Build history of the part. All positions in model axes, mm. A direction names the side the tool comes from. Give positions to 0.01 mm unless a question says otherwise; leave off trailing zeros. Order: outer loops, then holes, each group sorted by start corner. A loop starts at its lowest first (then second) coordinate and runs counter-clockwise, first axis right, second up. Notation, with made-up numbers: (-16, -27) - (-2, -27) arc R8 cw to (-2, -13) - close; hole circle Ø2 at (-19.5, 45.5). An arc over 180 degrees is marked (long way). Write each question's results on one line, items separated by ' | '. Start each with the question number.
from build123d import *

# Parameters (mm, degrees)
PAD026_DEPTH    = 5
SKETCH058_R     = 2
POCKET036_DEPTH = 5.001
CHAMFER020_SIZE = 2


with BuildPart() as part:
    # Sketch053 → Pad026 (new body)
    with BuildSketch(Plane.XY):
        with BuildLine():
            Line((-81.323184, -45.417713), (-81.323184, -107.8))
            Line((-81.323184, -107.8), (-105.823184, -107.8))
            Line((-105.823184, -107.8), (-105.823184, 216.2))
            Line((-105.823184, 216.2), (-81.323184, 216.2))
            Line((-81.323184, 216.2), (-81.323184, -27.417713))
            Line((-89.323184, -27.417713), (-81.323184, -27.417713))
            ThreePointArc((-89.323184, -27.417713), (-98.323184, -36.417713), (-89.323184, -45.417713))
            Line((-89.323184, -45.417713), (-81.323184, -45.417713))
        make_face()
    extrude(amount=PAD026_DEPTH)

    # Sketch058 (on Face10 of Pad026) → Pocket036 (cut, through all)
    with BuildSketch(Plane.XY.offset(5)):
        with Locations((-99.573184, 211.2)):
            Circle(SKETCH058_R)
        with Locations((-87.573184, 211.2)):
            Circle(SKETCH058_R)
    extrude(amount=-POCKET036_DEPTH, mode=Mode.SUBTRACT)

    # Chamfer020
    chamfer020_edges = [part.edges().sort_by_distance(p)[0] for p in [
        (-89.573184, 211.2, 5),
        (-101.573184, 211.2, 5),
    ]]
    chamfer(chamfer020_edges, length=CHAMFER020_SIZE)


with BuildPart() as part_1:
    # Body019 placement: moved
    add(part.part.moved(Location((0, 0, 15.5))))


solid = part_1.part
Item 1: Flat gauge pin, fed straight in: pin 1 Ø3 at (x, y) = (-87.57, 211.2) entering from -Z. Where does the tip first touch, or does it go through?
Item 2: Probe line 1 along X through (y, z) = (211.2, 17.1); line 2 along Y through (x, z) = (-86.25, 20.3); line 3 along Y through (x, z) = (-90.5, 17.6). List the from-to ranges inside material, lowest first. Write a range as from..to.
Item 3: Which spindle directions (+Z, -Z, +X, -X, +Y, -Y) get a long thin tool onto all of the face, cutting with end or side? Do faces 1 (the flat face through (-93, 56, 15.5)), 2 (the flat face through (-85, -27.418, 18)). Say none if no direction does.
Item 4: Cut at A-A, the plane z = 16.55. List the corners of the cut face in (x, y).
Values found:
1) pin 1: passes through
2) line 1: x = -105.82..-101.57, -97.57..-89.57, -85.57..-81.32 | line 2: y = -107.8..-45.42, -27.42..207.64, 214.76..216.2 | line 3: y = -107.8..-45.34, -27.49..216.2
3) face 1: -Z, +X, -X, +Y, -Y | face 2: +Z, -Z, +X
4) outline: (-105.82, -107.8) - (-81.32, -107.8) - (-81.32, -45.42) - (-89.32, -45.42) arc R9 cw to (-89.32, -27.42) - (-81.32, -27.42) - (-81.32, 216.2) - (-105.82, 216.2) - close; hole circle Ø4 at (-99.57, 211.2); hole circle Ø4 at (-87.57, 211.2)
